```python
from build123d import *

# Parameters (mm, degrees)
SKETCH_1_W      = 60
SKETCH_1_H      = 120
EXTRUDE_1_DEPTH = 10
MM_1_D          = 5.5
MM_1_DEPTH      = 15
MM_1_TIP        = 1.652366702
MM_1_2_D        = 12
MM_1_2_DEPTH    = 15
MM_1_2_TIP      = 3.605163714


with BuildPart() as part:
    # 草图1 → 凸台-拉伸1 (new body)
    with BuildSketch(Plane.XY):
        Rectangle(SKETCH_1_W, SKETCH_1_H)
    extrude(amount=EXTRUDE_1_DEPTH)

    # mm _1
    with Locations(Plane(origin=(-15, -32, 10), x_dir=(1, 0, 0), z_dir=(0, 0, 1))):
        with Locations((0, 0), (30, 0), (30, -18), (0, -18)):
            Hole(MM_1_D / 2, depth=MM_1_DEPTH)
            with Locations((0, 0, -(MM_1_DEPTH + MM_1_TIP / 2))):  # 118° drill point
                Cone(0, MM_1_D / 2, MM_1_TIP, mode=Mode.SUBTRACT)

    # mm _1 2
    with Locations(Plane.XY.offset(10)):
        with Locations((-15, 30), (15, 30), (0, 50)):
            Hole(MM_1_2_D / 2, depth=MM_1_2_DEPTH)
            with Locations((0, 0, -(MM_1_2_DEPTH + MM_1_2_TIP / 2))):  # 118° drill point
                Cone(0, MM_1_2_D / 2, MM_1_2_TIP, mode=Mode.SUBTRACT)


solid = part.part
```
Can you work these out from the model? Positions are in its coordinate system, mm. Coordinates: 2 decimals unless noted, no trailing zeros. Order: outer loops, then holes, each group sorted by start corner. A loop starts at its lowest first (then second) coordinate and runs counter-clockwise, first axis right, second up. Notation, with made-up numbers: (62, -22.5) - (87, -22.5) arc R9 ccw to (87, -13.5) - close; hole circle Ø3 at (37.5, -32). An arc over 180 degrees is marked (long way). Answer in a Markdown table with one row per item.
1. If I drill on line 1 along Y through (x, z) = (15, 2.5); line 2 along Y through (x, z) = (0, 5.75); line 3 along Y through (x, z) = (12, 7.25), over which ranges is the centre line in solid material (lowest first)?
Reply:
| item | result |
|---|---|
| line 1 | y = -60 to -52.75, -47.25 to -34.75, -29.25 to 24, 36 to 60 |
| line 2 | y = -60 to 44, 56 to 60 |
| line 3 | y = -60 to 24.8, 35.2 to 60 |
2. Suppose I cut it at B-B (x = -15). Please give me the cut outline in (y, z), and give its area (3 significant figures).
Reply:
| item | result |
|---|---|
| outline | (-60, 0) - (-52.75, 0) - (-52.75, 10) - (-60, 10) - close; (-47.25, 0) - (-34.75, 0) - (-34.75, 10) - (-47.25, 10) - close; (-29.25, 0) - (24, 0) - (24, 10) - (-29.25, 10) - close; (36, 0) - (60, 0) - (60, 10) - (36, 10) - close |
| area | 970 mm^2 |
3. Suppose I cut it at C-C (z = 3.75). Please give me the cut outline in (x, y), and give its area (3 significant figures).
Reply:
| item | result |
|---|---|
| outline | (-30, -60) - (30, -60) - (30, 60) - (-30, 60) - close; hole circle Ø12 at (-15, 30); hole circle Ø5.5 at (-15, -50); hole circle Ø5.5 at (-15, -32); hole circle Ø12 at (0, 50); hole circle Ø12 at (15, 30); hole circle Ø5.5 at (15, -50); hole circle Ø5.5 at (15, -32) |
| area | 6,770 mm^2 |
4. For pin 1 (3.5 mm diameter, centred on x = 15, y = -50, fed in from -Z), with a flat end and sliding along its axis, tell me the tip position at first contact or that it passes through.
Reply:
| item | result |
|---|---|
| pin 1 | passes through |
5. Suppose I cut it at A-A (y = -50). Please give me the cut outline in (x, z), and give its area (3 significant figures).
Reply:
| item | result |
|---|---|
| outline | (-30, 0) - (-17.75, 0) - (-17.75, 10) - (-30, 10) - close; (-12.25, 0) - (12.25, 0) - (12.25, 10) - (-12.25, 10) - close; (17.75, 0) - (30, 0) - (30, 10) - (17.75, 10) - close |
| area | 490 mm^2 |
6. Suppose I cut it at D-D (x = 2). Please give me the cut outline in (y, z).
Reply:
| item | result |
|---|---|
| outline | (-60, 0) - (44.34, 0) - (44.34, 10) - (-60, 10) - close; (55.66, 0) - (60, 0) - (60, 10) - (55.66, 10) - close |
7. If we mould it in two halves opening along Y, with no side actions, what happens to faces 1 (the flat face through (0, 60, 5)), 2 (the flat face through (30, -1, 5)), 3 (the cylindrical face through (-14.642, -29.273, 4.93))? For each: pulls with the +Y half, pulls with the -Y half, needs draft (parallel to the pull), parting line crosses it, or undercut.
Reply:
| item | result |
|---|---|
| face 1 | pulls with the +Y half |
| face 2 | needs draft |
| face 3 | undercut |
